The model under review builds one solid part; all positions refer to its coordinate system, in mm. A direction names the side the tool comes from. Coordinates: 2 decimals unless noted, no trailing zeros. Loops run counter-clockwise (first coordinate to the right, second up) from the corner with the lowest first, then second, coordinate; pieces in that order, holes last. Notation, with made-up numbers: M 22.5,8.25 L 80.5,8.25 A16 ccw 80.5,25.25 Z; hole C 86.25,4 d9. An arc over 180 degrees is marked long. Write item = value, one per line. Start each with the question number.
Q1. Mouldability with a two-part tool opening along X and no side actions: class faces 3 (the face through (47.15, -3.01, 250.44)), 4 (the face through (20, 0, 250)), 5 (the face through (47, -30, 250)) as released by +X, released by -X, zero draft, split by the parting line, or undercut.
Q2. Wall thickness on probe 1 along Z at (x, y) = (21, -2.1); probe 2 along Y at (x, z) = (5.5, 59.5); probe 3 along X at (y, z) = (-17, 83): over which ranges is each line inside the solid? List them lowest first.
Q3. Clearance check with flat-ended pins moving along their axes: pin 1 Ø12 at (x, y) = (26.5, -11) entering from -Z; pin 2 Ø8 at (x, z) = (21, 84) entering from -Y; pin 3 Ø3 at (y, z) = (-12, 160.5) entering from -X. State where each tip first meets the part, or that it passes through.
Q4. We need section A-A on z = 443. Give the boundary of the cut face in (x, y).
Q5. For faces 1 (the face through (20, -3, 250)), 2 (the face through (36, -2.7, 508)), list the 3-axis set-ups (+Z, -Z, +X, -X, +Y, -Y) from which the entire face can be reached by the end or side of a thin tool; tool diameter is ignored.
Q6. We need section C-C on y = -41. Give the boundary of the cut face in (x, z), and give its area (3 significant figures).
Q7. We need section B-B on x = 8.5. Give the boundary of the cut face in (y, z), and give its area (3 significant figures).
from build123d import *

# Parameters (mm, degrees)
F1_DEPTH = 508
F2_R     = 3
F3_DEPTH = 50.001
F4_R     = 3
F5_DEPTH = 50.001


with BuildPart() as f1:
    # F0 (on Top) → F1 (new body)
    with BuildSketch(Plane.XY):
        with BuildLine():
            Line((40, 0), (0, 0))
            Line((0, 0), (0, -3))
            Line((0, -3), (40, -3))
            ThreePointArc((40, -3), (44.949747, -5.050253), (47, -10))
            Line((47, -10), (47, -50))
            Line((47, -50), (50, -50))
            Line((50, -50), (50, -10))
            ThreePointArc((50, -10), (47.071068, -2.928932), (40, 0))
        make_face()
    extrude(amount=F1_DEPTH)

    # F2 (on face) → F3 (cut, through all)
    with BuildSketch(Plane(origin=(0, 0, 0), x_dir=(-1, 0, 0), z_dir=(0, 1, 0))):
        with Locations((-21, 464)):
            Circle(F2_R)
        with Locations((-21, 274)):
            Circle(F2_R)
        with Locations((-21, 84)):
            Circle(F2_R)
    extrude(amount=-F3_DEPTH, mode=Mode.SUBTRACT)

    # F4 (on face) → F5 (cut, through all)
    with BuildSketch(Plane.YZ.offset(50)):
        with Locations((-29, 464)):
            Circle(F4_R)
        with Locations((-29, 274)):
            Circle(F4_R)
        with Locations((-29, 84)):
            Circle(F4_R)
    extrude(amount=-F5_DEPTH, mode=Mode.SUBTRACT)


solid = f1.part
Returned:
q1.face_3 = released by +X
q1.face_4 = zero draft
q1.face_5 = released by -X
q2.probe_1 = 0 to 81, 87 to 271, 277 to 461, 467 to 508
q2.probe_2 = -3 to 0
q2.probe_3 = 47 to 50
q3.pin_1 = through
q3.pin_2 = -3
q3.pin_3 = 47
q4.outline = M 0,-3 L 40,-3 A7 cw 47,-10 L 47,-50 L 50,-50 L 50,-10 A10 ccw 40,0 L 0,0 Z
q5.face_1 = +Z, -Z, -X, -Y
q5.face_2 = +Z, +X, -X, +Y, -Y
q6.outline = M 47,0 L 50,0 L 50,508 L 47,508 Z
q6.area = 1,520 mm^2
q7.outline = M -3,0 L 0,0 L 0,508 L -3,508 Z
q7.area = 1,520 mm^2
